For this review, take the finished solid that the model builds, in its own axes (mm). A direction names the side the tool comes from. Coordinates: 2 decimals unless noted, no trailing zeros. Loops run counter-clockwise (first coordinate to the right, second up) from the corner with the lowest first, then second, coordinate; pieces in that order, holes last. Notation, with made-up numbers: M 48.25,83.5 L 57.25,83.5 A26 ccw 57.25,106.5 Z; hole C -23.75,7.25 d4. An arc over 180 degrees is marked long. Put each result on its own line as item: value.
```python
from build123d import *

# Parameters (mm, degrees)
BOSS_EXTRUDE1_DEPTH          = 2.5
BOSS_EXTRUDE2_DEPTH          = 12
F_4_0_4_DIAMETER_HOLE1_D     = 4
F_4_0_4_DIAMETER_HOLE2_D     = 4
F_5_2_5_2_DIAMETER_HOLE1_D   = 5.2
CHAMFER5_SIZE                = 8.5
FILLET13_R                   = 6
CHAMFER1_SIZE                = 5
CHAMFER2_SIZE                = 1
CHAMFER4_SIZE                = 0.8
CUT_REVOLVE1_ANGLE           = 60
CUT_REVOLVE1_OTHER_WAY_ANGLE = 60
FILLET4_R                    = 1
FILLET5_R                    = 8
FILLET6_R                    = 3
FILLET7_R                    = 2
FILLET11_R                   = 5
FILLET12_R                   = 2
CUT_EXTRUDE2_DEPTH           = 38
CHAMFER8_SIZE                = 6.868693549
CHAMFER8_SIZE_2              = 2.5
FILLET14_R                   = 3
M3_CLEARANCE_HOLE1_D         = 3.4


with BuildPart() as part:
    # Sketch1 → Boss-Extrude1 (new body)
    with BuildSketch(Plane(origin=(0, 0, 0), x_dir=(1, 0, 0), z_dir=(0, 1, 0))):
        with BuildLine():
            Line((-7.904447763, 6.416984589), (-51.546411114, 0.671411114))
            ThreePointArc((-51.546411114, 0.671411114), (-51.035673477, -0.364262362), (-50, -0.875))
            Line((-50, -0.875), (-0.965087675, -7.330568677))
            ThreePointArc((-0.965087675, -7.330568677), (3.516208172, -6.504222585), (6.661937904, -3.207368814))
            Line((6.661937904, -3.207368814), (21.2, 26.989241728))
            Line((21.2, 26.989241728), (2, 26.989241728))
            Line((2, 26.989241728), (-7.904447763, 6.416984589))
        make_face()
    extrude(amount=BOSS_EXTRUDE1_DEPTH)

    # Sketch1<6> → Boss-Extrude2 (add)
    with BuildSketch(Plane(origin=(0, 0, 0), x_dir=(1, 0, 0), z_dir=(0, 1, 0))):
        Polygon((2, 42), (2, 26.989241728), (68.2, 26.989241728), (68.2, 38.789241728), (15.919770539, 38.789241728), (12, 32), (7, 32), (7, 42), align=None)
    extrude(amount=BOSS_EXTRUDE2_DEPTH)

    # Ø4.0 (4) Diameter Hole1 (through all)
    with Locations(Plane(origin=(0, 0, 0), x_dir=(-1, 0, 0), z_dir=(0, -1, 0))):
        with Locations((-57.170705016, 32.889241728), (-33.229294984, 32.889241728)):
            Hole(F_4_0_4_DIAMETER_HOLE1_D / 2)

    # Ø4.0 (4) Diameter Hole2 (through all)
    with Locations(Plane(origin=(0, 0, 0), x_dir=(-1, 0, 0), z_dir=(0, -1, 0))):
        with Locations((0, 0)):
            Hole(F_4_0_4_DIAMETER_HOLE2_D / 2)

    # Ø5.2 (5.2) Diameter Hole1 (through all)
    with Locations(Plane(origin=(0, 0, 0), x_dir=(-1, 0, 0), z_dir=(0, -1, 0))):
        with Locations((-45.2, 32.889241728)):
            Hole(F_5_2_5_2_DIAMETER_HOLE1_D / 2)

    # Chamfer5
    chamfer5_edges = [part.edges().sort_by_distance(p)[0] for p in [
        (11.6, 2.5, -26.989241728),
    ]]
    chamfer(chamfer5_edges, length=CHAMFER5_SIZE)

    # Fillet13
    fillet13_edges = [part.edges().sort_by_distance(p)[0] for p in [
        (21.2, 5.5, -26.989241728),
    ]]
    fillet(fillet13_edges, radius=FILLET13_R)

    # Chamfer1
    chamfer1_edges = [part.edges().sort_by_distance(p)[0] for p in [
        (68.2, 0, -32.889241728),
        (68.2, 6, -26.989241728),
        (68.2, 6, -38.789241728),
        (68.2, 12, -32.889241728),
    ]]
    chamfer(chamfer1_edges, length=CHAMFER1_SIZE)

    # Chamfer2
    # the kernel refuses this chamfer: 1 mm, written as the material it takes off along each edge
    with BuildSketch(Plane(origin=(24.970484005, 0, -26.989241728), x_dir=(0, 0, -1), z_dir=(1, 0, 0))) as chamfer2_piece_1:
        Polygon((CHAMFER2_SIZE, 0), (0, CHAMFER2_SIZE), (0, 0), align=None)
    extrude(amount=40.801198983, mode=Mode.SUBTRACT)
    with BuildSketch(Plane(origin=(-0.571682988, 12, -26.989241728), x_dir=(0, -1, 0), z_dir=(1, 0, 0))) as chamfer2_piece_2:
        Polygon((CHAMFER2_SIZE, 0), (0, CHAMFER2_SIZE), (0, 0), align=None)
    extrude(amount=66.343365976, mode=Mode.SUBTRACT)
    with BuildSketch(Plane(origin=(65.771682988, 12, -38.789241728), x_dir=(0, -1, 0), z_dir=(-1, 0, 0)), Plane(origin=(65.771682988, 0, -38.789241728), x_dir=(0, 0, 1), z_dir=(-1, 0, 0))) as chamfer2_piece_3:
        Polygon((CHAMFER2_SIZE, 0), (0, CHAMFER2_SIZE), (0, 0), align=None)
    extrude(amount=52.423595437, mode=Mode.SUBTRACT)
    with BuildSketch(Plane(origin=(24.970484005, 0, -20.989241728), x_dir=(-0.9610284466527214, -1.1097335043339142e-15, 0.27644949760174536), z_dir=(0.27644949760174536, 0, 0.9610284466527214))) as chamfer2_piece_4:
        Polygon((6 + CHAMFER2_SIZE, 0), (6, -CHAMFER2_SIZE), (6, 0), align=None)
    revolve(axis=Axis((24.970484005, 0, -20.989241728), (0, -1, 0)), revolution_arc=106.048413393, mode=Mode.SUBTRACT)

    # Chamfer4
    # the kernel refuses this chamfer: 0.8 mm, written as the material it takes off along each edge
    with BuildSketch(Plane(origin=(62.505076275, -0.694923725, -39.484165453), x_dir=(-0.40824829046386635, -0.4082482904638597, 0.816496580927726), z_dir=(0.5773502691896258, 0.5773502691896258, 0.5773502691896258)), Plane(origin=(62.505076275, 12.694923725, -39.484165453), x_dir=(-0.40824829046386746, -0.816496580927726, -0.4082482904638586), z_dir=(0.5773502691896258, -0.5773502691896258, 0.5773502691896258)), Plane(origin=(69.394923725, 5.805076275, -33.184165453), x_dir=(-0.408248290463863, -0.816496580927726, 0.408248290463863), z_dir=(-0.5773502691896258, 0.5773502691896258, 0.5773502691896258))) as chamfer4_piece_1:
        Polygon((CHAMFER4_SIZE, 0), (-CHAMFER4_SIZE * 0.5, -CHAMFER4_SIZE * 0.866025403784), (0, 0), align=None)
    extrude(amount=11.933565841, mode=Mode.SUBTRACT)
    with BuildSketch(Plane(origin=(62.505076275, -0.694923725, -26.294318002), x_dir=(-0.4082482904638641, -0.4082482904638619, -0.816496580927726), z_dir=(0.5773502691896258, 0.5773502691896258, -0.5773502691896258))) as chamfer4_piece_2:
        Polygon((CHAMFER4_SIZE, 0), (-CHAMFER4_SIZE * 0.5, CHAMFER4_SIZE * 0.866025403784), (0, 0), align=None)
    extrude(amount=11.933565841, mode=Mode.SUBTRACT)

    # Sketch7 → Cut-Revolve1 (revolve, cut)
    with BuildSketch(Plane.XY.offset(-32.889241728)):
        Polygon((68.2, 6.920204103), (60.2, 12), (60.2, 14), (68.2, 14), align=None)
    revolve(axis=Axis((68.2, 6.920204103, -32.889241728), (-0.8441922430161829, 0.5360405365560577, 0)), revolution_arc=CUT_REVOLVE1_ANGLE, mode=Mode.SUBTRACT)

    # Sketch7 → Cut-Revolve1 other way (revolve, cut)
    with BuildSketch(Plane.XY.offset(-32.889241728)):
        Polygon((68.2, 6.920204103), (60.2, 12), (60.2, 14), (68.2, 14), align=None)
    revolve(axis=Axis((68.2, 6.920204103, -32.889241728), (0.8441922430161829, -0.5360405365560577, 0)), revolution_arc=CUT_REVOLVE1_OTHER_WAY_ANGLE, mode=Mode.SUBTRACT)

    # Fillet4
    # the kernel refuses this fillet: 1 mm, written as the material it adds along each edge
    with BuildSketch(Plane(origin=(69.418486547, 6.146496233, -32.889241728), x_dir=(0.26802026827802927, 0.42209612150809256, -0.8660254037844378), z_dir=(-0.8441922430161831, 0.5360405365560573, 0))) as fillet4_piece_1_section:
        with BuildLine():
            CenterArc((FILLET4_R * 0.57735026919, -FILLET4_R), FILLET4_R, 90, 60)
            Line((-FILLET4_R * 0.288675134595, -FILLET4_R * 0.5), (0, 0))
            Line((0, 0), (FILLET4_R * 0.57735026919, 0))
        make_face()
    fillet4_piece_1 = extrude(amount=12.363265808, mode=Mode.PRIVATE)
    fillet4_piece_1 = split(fillet4_piece_1, bisect_by=Plane(origin=(69.418486547, 12, -32.889241728), z_dir=(0, -1, 0)), keep=Keep.TOP, mode=Mode.PRIVATE)
    fillet4_piece_1 = split(fillet4_piece_1, bisect_by=Plane(origin=(68.864064806, 5.869285362, -33.166452598), z_dir=(-0.8164965809277263, -0.4082482904637079, -0.4082482904640183)), keep=Keep.TOP, mode=Mode.PRIVATE)
    fillet4_piece_1 = split(fillet4_piece_1, bisect_by=Plane(origin=(69.235995157, 5.964004843, -32.889241728), z_dir=(-0.7071067811865476, -0.7071067811865476, 0)), keep=Keep.TOP, mode=Mode.PRIVATE)
    fillet4_piece_1 = split(fillet4_piece_1, bisect_by=Plane(origin=(68.864064806, 5.869285362, -32.612030857), z_dir=(-0.8164965809277263, -0.4082482904637079, 0.4082482904640183)), keep=Keep.TOP, mode=Mode.PRIVATE)
    add(fillet4_piece_1)

    # Fillet5
    fillet5_edges = [part.edges().sort_by_distance(p)[0] for p in [
        (7.507702037, 2.5, -18.489241728),
        (-7.904447763, 1.25, -6.416984589),
        (2, 5.5, -26.989241728),
    ]]
    fillet(fillet5_edges, radius=FILLET5_R)

    # Fillet6
    fillet6_edges = [part.edges().sort_by_distance(p)[0] for p in [
        (15.919770539, 6, -38.789241728),
        (12, 6, -32),
    ]]
    fillet(fillet6_edges, radius=FILLET6_R)

    # Fillet7
    fillet7_edges = [part.edges().sort_by_distance(p)[0] for p in [
        (7, 6, -32),
    ]]
    fillet(fillet7_edges, radius=FILLET7_R)

    # Fillet11
    fillet11_edges = [part.edges().sort_by_distance(p)[0] for p in [
        (4.5, 0, -42),
        (4.5, 12, -42),
    ]]
    fillet(fillet11_edges, radius=FILLET11_R)

    # Fillet12
    # the kernel refuses this fillet: 2 mm, written as the material it takes off along each edge
    with BuildSketch(Plane(origin=(2, 0, -42), x_dir=(0, 0, 1), z_dir=(0, 1, 0))) as fillet12_piece_1:
        with BuildLine():
            CenterArc((FILLET12_R, FILLET12_R), FILLET12_R, 180, 90)
            Line((0, FILLET12_R), (0, 0))
            Line((0, 0), (FILLET12_R, 0))
        make_face()
    extrude(amount=12, mode=Mode.SUBTRACT)
    with BuildSketch(Plane(origin=(7, 0, -42), x_dir=(0, 0, 1), z_dir=(0, 1, 0))) as fillet12_piece_2:
        with BuildLine():
            CenterArc((FILLET12_R, -FILLET12_R), FILLET12_R, 90, 90)
            Line((0, -FILLET12_R), (0, 0))
            Line((0, 0), (FILLET12_R, 0))
        make_face()
    extrude(amount=12, mode=Mode.SUBTRACT)

    # Sketch11 → Cut-Extrude2 (cut)
    with BuildSketch(Plane(origin=(-50.581323439, 0, 6.659157562), x_dir=(0, -1, 0), z_dir=(0.9914448613738103, 0, -0.1305261922200527))):
        Polygon((-2, 7.393823865), (0, 1.898869026), (0, 7.393823865), align=None)
    extrude(amount=CUT_EXTRUDE2_DEPTH, mode=Mode.SUBTRACT)

    # Chamfer8
    # the kernel refuses this chamfer: 6.868693549, 2.5 mm, written as the material it takes off along each edge
    with BuildSketch(Plane(origin=(-10.828460053, 0, 17.48282525), x_dir=(0.9914448613738103, 0, -0.1305261922200527), z_dir=(-0.1305261922200527, 0, -0.9914448613738103))) as chamfer8_piece_1_section:
        Polygon((CHAMFER8_SIZE, 0), (0, -CHAMFER8_SIZE_2), (0, 0), align=None)
    chamfer8_piece_1 = extrude(amount=41.132412086, mode=Mode.PRIVATE)
    chamfer8_piece_1 = split(chamfer8_piece_1, bisect_by=Plane(origin=(-11.100528233, -5.72682899, 15.416262251), z_dir=(-0.04464258697085675, -0.939692620785907, -0.3390941135865724)), keep=Keep.TOP, mode=Mode.PRIVATE)
    add(chamfer8_piece_1, mode=Mode.SUBTRACT)

    # Fillet14
    fillet14_edges = [part.edges().sort_by_distance(p)[0] for p in [
        (-9.426930062, 1, -3.445360698),
    ]]
    fillet(fillet14_edges, radius=FILLET14_R)

    # M3 Clearance Hole1 (through all)
    with Locations(Plane(origin=(0, 2.5, 0), x_dir=(1, 0, 0), z_dir=(0, 1, 0))):
        with Locations((0.467987162, 12.175533229), (8.467987162, 12.175533229)):
            Hole(M3_CLEARANCE_HOLE1_D / 2)


solid = part.part
```
(1) Add section A-A (x = 45.2). Write out the cut boundary in (y, z).
Determined:
outline: M 0,-37.79 L 1,-38.79 L 11,-38.79 L 12,-37.79 L 12,-35.49 L 0,-35.49 Z; M 0,-30.29 L 12,-30.29 L 12,-27.99 L 11,-26.99 L 1,-26.99 L 0,-27.99 Z
(2) Add section C-C (x = -26.5). Write out the cut boundary in (y, z), plus the area to 3 significant figures.
Determined:
outline: M 0,1.57 L 2,-3.97 L 2.5,-3.97 L 2.5,3.97 L 0,3.97 Z
area: 14.3 mm^2
(3) Draft analysis for pull direction Z (two halves, no side actions). For faces 1 (the flat face through (63.904, 10.479, -31.673)), 2 (the flat face through (65.11, 5.93, -28.9)), 3 (the flat face through (41, 6, -38.789)), 4 (the flat face through (65.5, 9.7, -34.7)), state which applies: +Z half, -Z half, draft (parallel to the pull), parting line (faces both ways), or undercut.
Determined:
face 1: undercut
face 2: +Z half
face 3: -Z half
face 4: draft
(4) Add section D-D (x = -40). Write out the cut boundary in (y, z), plus the area to 3 significant figures.
Determined:
outline: M 0.42,2.19 L 2,-2.19 L 2.5,-2.19 L 2.5,2.19 Z
area: 5.66 mm^2
(5) Add section B-B (x = 28). Write out the cut boundary in (y, z), plus the area to 3 significant figures.
Determined:
outline: M 0,-37.79 L 1,-38.79 L 11,-38.79 L 12,-37.79 L 12,-27.99 L 11,-26.99 L 1,-26.99 L 0,-27.99 Z
area: 140 mm^2
(6) Tool access review of faces 5 (the cylindrical face through (-7.821, 1.545, -7.896)), 6 (the cylindrical face through (16.133, 6.084, -38.376)), 7 (the cylindrical face through (-9.859, 1.043, -3.764)): name each direction out of +Z, -Z, +X, -X, +Y, -Y from which nothing blocks a thin tool from reaching the whole face with its end or side.
Determined:
face 5: -Z, -X, +Y, -Y
face 6: -Z, +Y, -Y
face 7: -X, -Y
(7) Wall thickness on line 1 along Z through (x, y) = (31, 1.5); line 2 along X through (y, z) = (3.75, -30.5); line 3 along Z through (x, y) = (11, 5.75): over which ranges is each line inside the solid? List them lowest first. Write a range as [from, to].
Determined:
line 1: z = [-38.79, -26.99]
line 2: x = [2, 44.17], [46.23, 66.34]
line 3: z = [-32.09, -21.74]
(8) For pin 1 (3.5 mm diameter, centred on y = 5.5, z = -33.5, fed in from -X); pin 2 (5 mm diameter, centred on x = -15, y = 7, fed in from -Z); pin 3 (3 mm diameter, centred on x = 36, y = 4.5, fed in from -Z); pin 4 (5.5 mm diameter, centred on x = 0.47, z = -12.18, fed in from +Y), all flat-tipped, find the tip position at first contact; note any pin that passes through.
Determined:
pin 1: stops at x = 2
pin 2: passes through
pin 3: stops at z = -38.79
pin 4: stops at y = 2.5
